Here's how the part is built. I have some questions about the finished solid (model axes, mm). Face numbers are marked on the shaded views. A direction names the side the tool comes from. Round coordinates to 2 decimals unless told otherwise and drop trailing zeros. Loops run counter-clockwise (first coordinate to the right, second up) from the corner with the lowest first, then second, coordinate; pieces in that order, holes last. Notation, with made-up numbers: M 0.5,39.25 L 41.5,39.25 A22 ccw 41.5,53.25 Z; hole C -3.75,30 d3. An arc over 180 degrees is marked long. Put each result on its own line as item: value. Start each with the question number.
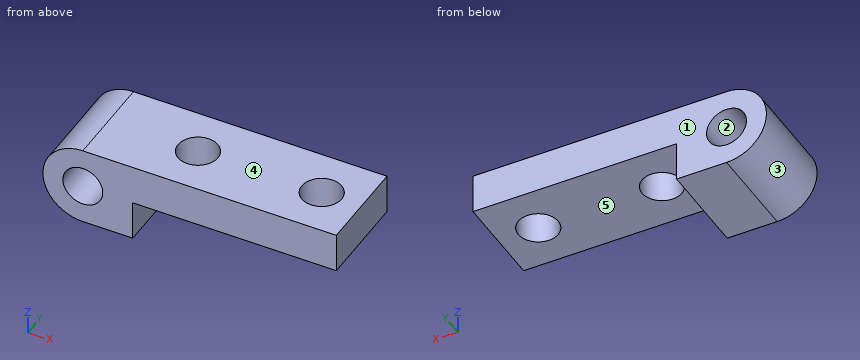
Autodesk Inventor part; units mm, degrees
ref_plane "YZ Plane" through (0, 0, 0) normal (1, 0, 0) x (0, 1, 0)
ref_plane "XZ Plane" through (0, 0, 0) normal (0, 1, 0) x (-1, 0, 0)
ref_plane "XY Plane" through (0, 0, 0) normal (0, 0, 1) x (1, 0, 0)
ref_plane "Work Plane1" through (-181, -1, -216) normal (0, 1, 0) x (-1, 0, 0)
sketch "Sketch1" plane through (-181, -1, -216) normal (0, 1, 0) x (-1, 0, 0)
  circle A0 centre (-9, -5) radius 2
  arc A1 (-18, -6.825) -> (-14.825, -10) centre (-14.825, -6.825) ccw
  line L0 (-3.175, -10) -> (-14.825, -10)
  arc A2 (-3.175, -10) -> (0, -6.825) centre (-3.175, -6.825) ccw
  line L1 (0, -3.175) -> (0, -6.825)
  arc A3 (3.175, 0) -> (0, -3.175) centre (3.175, -3.175) ccw
  line L2 (-21.175, 0) -> (3.175, 0)
  arc A4 (-18, -3.175) -> (-21.175, 0) centre (-21.175, -3.175) ccw
  line L3 (-18, -3.175) -> (-18, -6.825)
  circle A5 centre (-9, -5) radius 5
  circle A6 centre (-9, -5) radius 4
  line L4 (-9, -1) -> (-34.4, -1)
  line L5 (-34.4, -1) -> (-34.4, -5)
  line L6 (-34.4, -5) -> (-14, -5)
  line L7 (-14, -5) -> (-14, -9)
  line L8 (-14, -9) -> (-9, -9)
  point P0 (-181, 216)
  dimension "d0" = 1
  dimension "d1" = 5
  dimension "d2" = 25.4
extrude "Extrusion1" add sketch "Sketch1" along normal blind 9.5 contours L6 L5 L4 A4 L3 | L3 A4 L4 A5 L6 | A5 L4 A6 L8 | A5 L8 L7 | A6 picked at (-12.1637, -8.3993)
sketch "Sketch2" plane through (-146.6, -1, -221) normal (0, 0, -1) x (-1, 0, 0)
  line L0 (0, 0) -> (20.4, 0)
  line L1 (20.4, 0) -> (20.4, 9.5)
  line L2 (0, 9.5) -> (20.4, 9.5)
  line L3 (0, 0) -> (0, 9.5)
  circle A0 centre (4, 4.75) radius 2
  circle A1 centre (16.4, 4.75) radius 2
  point P0 (-146.6, 1)
  dimension "d5" = 4
  dimension "d6" = 4
  dimension "d7" = 4
  dimension "d8" = 4
  dimension "d9" = 4.75
  dimension "d10" = 4.75
extrude "Extrusion2" cut sketch "Sketch2" against normal blind 9.5 contours A0 | A1
properties part number "flappythingadaptor"
1) On a 3-axis mill with a long thin cutter (end or side, diameter ignored), from which of +Z, -Z, +X, -X, +Y, -Y can I reach the whole of each face in a straight line? I mean the marked faces 4 and 5. Say none if no direction works.
2) If we mould it in two halves opening along Z, with no side actions, what happens to the marked faces 1, 2 and 3? For each: pulls with the +Z half, pulls with the -Z half, needs draft (parallel to the pull), parting line crosses it, or undercut.
3) If I drill on probe 1 along Y at (x, z) = (-150.6, -219.65); probe 2 along X at (y, z) = (4.25, -217.5); probe 3 along Z at (x, y) = (-172, 6.25), over which ranges is the centre line in solid material (lowest first)? Write a range as from..to.
4) Suppose I cut it at B-B (z = -220). Write out the boundary of the cut face in (x, y).
5) Suppose I cut it at C-C (x = -150.6). Write out the boundary of the cut face in (y, z), plus the area to 3 significant figures.
6) Suppose I cut it at D-D (y = 3.25). Write out the boundary of the cut face in (x, z), plus the area to 3 significant figures.
7) Suppose I cut it at A-A (y = 1). Write out the boundary of the cut face in (x, z).
8) I'm going to push flat-ended pins straight in: P1, Ø1, axis at x = -155, z = -222, coming from the +Y side; P2, Ø5, axis at x = -163, y = 3.75, coming from the +Z side; P3, Ø1.5, axis at y = 1.5, z = -222.5, coming from the -X side; P4, Ø2, axis at y = 2.5, z = -222.5, coming from the +X side. Where does each tip first touch, or does it pass through?
Results are:
1. face 4: +Z, +X, -X, +Y, -Y
1. face 5: -Z, +X, +Y, -Y
2. face 1: needs draft
2. face 2: undercut
2. face 3: parting line crosses it
3. probe 1: -1..1.75, 5.75..8.5
3. probe 2: -173.94..-164.94, -161.06..-152.54, -148.66..-146.6
3. probe 3: -225..-223, -219..-217
4. outline: M -175.87,-1 L -173.73,-1 L -173.73,8.5 L -175.87,8.5 Z; M -170.27,-1 L -146.6,-1 L -146.6,8.5 L -170.27,8.5 Z; hole C -163,3.75 d4; hole C -150.6,3.75 d4
5. outline: M -1,-221 L 1.75,-221 L 1.75,-217 L -1,-217 Z; M 5.75,-221 L 8.5,-221 L 8.5,-217 L 5.75,-217 Z
5. area: 22.0 mm²
6. outline: M -172,-225 L -167,-225 L -167,-221 L -164.94,-221 L -164.94,-217 L -172,-217 A4 ccw Z; M -161.06,-221 L -152.54,-221 L -152.54,-217 L -161.06,-217 Z; M -148.66,-221 L -146.6,-221 L -146.6,-217 L -148.66,-217 Z; hole C -172,-221 d4
6. area: 103 mm²
7. outline: M -172,-225 L -167,-225 L -167,-221 L -146.6,-221 L -146.6,-217 L -172,-217 A4 ccw Z; hole C -172,-221 d4
8. P1: through
8. P2: z = -217
8. P3: x = -175.93
8. P4: x = -167
